```python
from build123d import *

# Parameters (mm, degrees)
SKETCH1_W             = 41
SKETCH1_H             = 5
SKETCH1_R             = 1
BOSS_EXTRUDE1_DEPTH   = 10
CUT_EXTRUDE1_DEPTH    = 10
SKETCH4_W             = 38
SKETCH4_H             = 15
BOSS_EXTRUDE2_DEPTH   = 0.7
SKETCH3_W             = 26.4
SKETCH3_H             = 3.8
CUT_EXTRUDE2_DEPTH    = 10
CHAMFER1_SIZE         = 3
CHAMFER1_SIZE2        = 0.803847577
CHAMFER1_PART_2_SIZE  = 3
CHAMFER1_PART_2_SIZE2 = 0.803847577
CHAMFER1_PART_3_SIZE  = 3
CHAMFER1_PART_3_SIZE2 = 0.803847577
SKETCH7_W             = 26.4
SKETCH7_H             = 3.8
BOSS_EXTRUDE3_DEPTH   = 0.8


with BuildPart() as part:
    # Sketch1 → Boss-Extrude1 (new body)
    with BuildSketch(Plane(origin=(0, 0, 0), x_dir=(1, 0, 0), z_dir=(0, 1, 0))):
        with Locations((20.5, 2.5)):
            Rectangle(SKETCH1_W, SKETCH1_H)
        with Locations((1.5, 1.5)):
            Circle(SKETCH1_R, mode=Mode.SUBTRACT)
        with Locations((39.5, 1.5)):
            Circle(SKETCH1_R, mode=Mode.SUBTRACT)
    extrude(amount=BOSS_EXTRUDE1_DEPTH)

    # Sketch2 → Cut-Extrude1 (cut)
    with BuildSketch(Plane.XY):
        Polygon((0, 10), (0, 1.2), (9, 1.2), (9, 4.6), (37, 4.6), (37, 1.2), (41, 1.2), (41, 10), align=None)
    extrude(amount=-CUT_EXTRUDE1_DEPTH, mode=Mode.SUBTRACT)

    # Sketch4 → Boss-Extrude2 (add)
    with BuildSketch(Plane(origin=(0, 0, -5), x_dir=(-1, 0, 0), z_dir=(0, 0, -1))):
        with Locations((-22, 7.5)):
            Rectangle(SKETCH4_W, SKETCH4_H)
    extrude(amount=BOSS_EXTRUDE2_DEPTH)

    # Sketch3 → Cut-Extrude2 (cut)
    with BuildSketch(Plane.XY):
        with Locations((23, 1.9)):
            Rectangle(SKETCH3_W, SKETCH3_H)
    extrude(amount=-CUT_EXTRUDE2_DEPTH, mode=Mode.SUBTRACT)

    # Chamfer1
    chamfer1_edges = [part.edges().sort_by_distance(p)[0] for p in [
        (37, 1.2, -2.5),
    ]]
    chamfer1_side = [part.faces().sort_by_distance(p)[0] for p in [
        (37, 2.9, -2.5),
    ]]
    chamfer(chamfer1_edges, length=CHAMFER1_SIZE, length2=CHAMFER1_SIZE2, reference=chamfer1_side[0])

    # Chamfer1 part 2
    chamfer1_part_2_edges = [part.edges().sort_by_distance(p)[0] for p in [
        (9, 1.2, -2.5),
    ]]
    chamfer1_part_2_side = [part.faces().sort_by_distance(p)[0] for p in [
        (9, 2.9, -2.5),
    ]]
    chamfer(chamfer1_part_2_edges, length=CHAMFER1_PART_2_SIZE, length2=CHAMFER1_PART_2_SIZE2, reference=chamfer1_part_2_side[0])

    # Chamfer1 part 3
    chamfer1_part_3_edges = [part.edges().sort_by_distance(p)[0] for p in [
        (39, 1.2, -5),
        (6, 1.2, -5),
    ]]
    chamfer1_part_3_side = [part.faces().sort_by_distance(p)[0] for p in [
        (21.778191985, 9.253401678, -5),
    ]]
    chamfer(chamfer1_part_3_edges, length=CHAMFER1_PART_3_SIZE, length2=CHAMFER1_PART_3_SIZE2, reference=chamfer1_part_3_side[0])

    # Sketch7 → Boss-Extrude3 (add)
    with BuildSketch(Plane.XY):
        with Locations((23, 1.9)):
            Rectangle(SKETCH7_W, SKETCH7_H)
    extrude(amount=-BOSS_EXTRUDE3_DEPTH)


solid = part.part
```
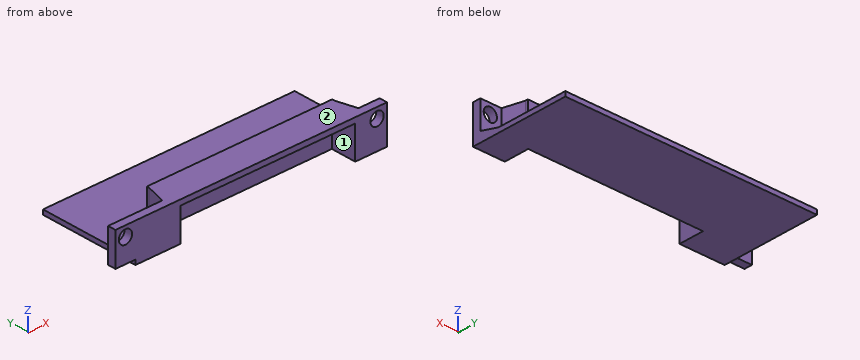
Model file for the job. Use its own axes, mm. Face numbers are marked on the shaded views. Coordinates: 2 decimals unless noted, no trailing zeros. Loops run counter-clockwise (first coordinate to the right, second up) from the corner with the lowest first, then second, coordinate; pieces in that order, holes last. Notation, with made-up numbers: M 33.5,37 L 89.5,37 A32 cw 89.5,73 Z; hole C -39,-29.75 d6. An arc over 180 degrees is marked long. Use CSV: the item, a comma, the result in double quotes. Start each with the question number.
1. Band-saw the part on B-B, the plane x = 1.5. List the corners of the cut face in (y, z), then the cut area to 3 significant figures.
2. Probe probe 1 along X at (y, z) = (0.35, -1.5); probe 2 along Z at (x, y) = (39.5, 0.45); probe 3 along Z at (x, y) = (1.5, 0.75). List the from-to ranges inside material, lowest first. Write a range as [from, to].
3. Flat gauge pins, fed straight in: pin 1 (3 mm diameter, centred on x = 28, y = 1.5, fed in from -Z); pin 2 (3 mm diameter, centred on x = 20.5, y = 10, fed in from +Z); pin 3 (0.5 mm diameter, centred on y = 8, z = -5.5, fed in from -X). Where does each tip first touch, or does it go through?
4. Band-saw the part on A-A, the plane z = -1.5. List the corners of the cut face in (x, y).
5. Two-plate mould, pull along X, no slides. Class the marked faces 1 and 2: pulls with the +X half, pulls with the -X half, needs draft (parallel to the pull), parting line crosses it, or undercut.
6. Band-saw the part on D-D, the plane x = 39.5. List the corners of the cut face in (y, z), then the cut area to 3 significant figures.
7. Band-saw the part on C-C, the plane x = 14. List the corners of the cut face in (y, z).
Entries:
1,outline,"M 0,-5 L 1.2,-5 L 1.2,-2.5 L 0,-2.5 Z; M 0,-0.5 L 1.2,-0.5 L 1.2,0 L 0,0 Z"
1,area,"3.60 mm2"
2,probe 1,"x = [0, 0.5], [2.5, 9.8], [36.2, 38.5], [40.5, 41]"
2,probe 2,"z = [-5.7, -2.5], [-0.5, 0]"
2,probe 3,"z = [-5, -2.5], [-0.5, 0]"
3,pin 1,"stops at z = -0.8"
3,pin 2,"stops at z = -5"
3,pin 3,"stops at x = 3"
4,outline,"M 0,0 L 0.5,0 L 0.5,1.2 L 0,1.2 Z; M 2.5,0 L 9.8,0 L 9.8,3.8 L 36.2,3.8 L 36.2,0 L 38.5,0 L 38.5,1.2 L 37.8,1.2 L 37,4.2 L 37,4.6 L 9,4.6 L 9,4.2 L 8.2,1.2 L 2.5,1.2 Z; M 40.5,0 L 41,0 L 41,1.2 L 40.5,1.2 Z"
5,face 1,"undercut"
5,face 2,"needs draft"
6,outline,"M 0,-5.7 L 15,-5.7 L 15,-5 L 4.2,-5 L 1.2,-4.2 L 1.2,-2.5 L 0,-2.5 Z; M 0,-0.5 L 1.2,-0.5 L 1.2,0 L 0,0 Z"
6,area,"15.3 mm2"
7,outline,"M 0,-0.8 L 3.8,-0.8 L 3.8,-5.7 L 15,-5.7 L 15,-5 L 4.6,-5 L 4.6,0 L 0,0 Z"
